```python
from build123d import *

# Parameters (mm, degrees)
F0_R           = 12.7
F1_DEPTH       = 60.325
F2_DEPTH       = 25.4
F4_DEPTH       = 19.05
F5_DEPTH       = 41.275
F6_R           = 5.08
F7_R           = 6.35
F8_DEPTH       = 25.4
F9_W           = 44.704
F9_H           = 22.3266
F10_DEPTH      = 25.4
F10_DEPTH_BACK = 25.4


with BuildPart() as f1:
    # F0 (on Front) → F1 (new body)
    with BuildSketch(Plane.XZ):
        with BuildLine():
            Line((36.865121601, 0.0010602231), (-26.6348784242, 0.0010602231))
            ThreePointArc((-26.6348784242, 0.0010602231), (-64.8692857058, 15.7277157318), (-48.7691742678, -22.3509397769))
            Line((-48.7691742678, -22.3509397769), (43.0772257322, -22.3509397769))
            Line((43.0772257322, -22.3509397769), (36.865121601, 0.0010602231))
        make_face()
        with Locations((-48.986878399, 0)):
            Circle(F0_R, mode=Mode.SUBTRACT)
        Polygon((68.259521601, 0.0010602231), (36.865121601, 0.0010602231), (43.0772257322, -22.3509397769), (68.4772257322, -22.3509397769), align=None)
        with BuildLine():
            ThreePointArc((82.5471727442, 34.7990602231), (78.7429689335, 16.0288506516), (68.259521601, 0.0010602231))
            Line((68.259521601, 0.0010602231), (101.101721601, 0.0010602231))
            Line((101.101721601, 0.0010602231), (101.101721601, 34.7990602231))
            Line((101.101721601, 34.7990602231), (82.5471727442, 34.7990602231))
        make_face()
        Polygon((101.101721601, 0.0010602231), (68.259521601, 0.0010602231), (68.4772257322, -22.3509397769), (145.4392257322, -22.3509397769), (145.4392257322, 0.0010602231), (145.2215215758, 0.0010602231), align=None)
    extrude(amount=F1_DEPTH)

    # F0 (on Front) → F2 (join)
    with BuildSketch(Plane.XZ):
        with BuildLine():
            Line((36.865121601, 0.0010602231), (-26.6348784242, 0.0010602231))
            ThreePointArc((-26.6348784242, 0.0010602231), (-64.8692857058, 15.7277157318), (-48.7691742678, -22.3509397769))
            Line((-48.7691742678, -22.3509397769), (43.0772257322, -22.3509397769))
            Line((43.0772257322, -22.3509397769), (36.865121601, 0.0010602231))
        make_face()
        with Locations((-48.986878399, 0)):
            Circle(F0_R, mode=Mode.SUBTRACT)
        Polygon((68.259521601, 0.0010602231), (36.865121601, 0.0010602231), (43.0772257322, -22.3509397769), (68.4772257322, -22.3509397769), align=None)
        with BuildLine():
            ThreePointArc((82.5471727442, 34.7990602231), (78.7429689335, 16.0288506516), (68.259521601, 0.0010602231))
            Line((68.259521601, 0.0010602231), (101.101721601, 0.0010602231))
            Line((101.101721601, 0.0010602231), (101.101721601, 34.7990602231))
            Line((101.101721601, 34.7990602231), (82.5471727442, 34.7990602231))
        make_face()
        Polygon((101.101721601, 0.0010602231), (68.259521601, 0.0010602231), (68.4772257322, -22.3509397769), (145.4392257322, -22.3509397769), (145.4392257322, 0.0010602231), (145.2215215758, 0.0010602231), align=None)
    extrude(amount=F2_DEPTH)

    # F3 (on face) → F4 (cut)
    with BuildSketch(Plane.XZ.offset(60.325)):
        Polygon((68.259521601, 0.0010602231), (36.865121601, 0.0010602231), (43.0772257322, -22.3509397769), (68.4772257322, -22.3509397769), align=None)
    extrude(amount=-F4_DEPTH, mode=Mode.SUBTRACT)

    # F0 (on Front) → F5 (cut)
    with BuildSketch(Plane.XZ):
        with BuildLine():
            ThreePointArc((82.5471727442, 34.7990602231), (78.7429689335, 16.0288506516), (68.259521601, 0.0010602231))
            Line((68.259521601, 0.0010602231), (101.101721601, 0.0010602231))
            Line((101.101721601, 0.0010602231), (101.101721601, 34.7990602231))
            Line((101.101721601, 34.7990602231), (82.5471727442, 34.7990602231))
        make_face()
    extrude(amount=F5_DEPTH, mode=Mode.SUBTRACT)

    # F6
    f6_edges = [f1.edges().sort_by_distance(p)[0] for p in [
        (101.101722, -50.8, 34.79906),
    ]]
    fillet(f6_edges, radius=F6_R)

    # F7 (on face) → F8 (cut)
    with BuildSketch(Plane.XY.offset(0.0010602231)):
        with Locations((106.5772257322, -22.352)):
            Circle(F7_R)
    extrude(amount=-F8_DEPTH, mode=Mode.SUBTRACT)

    # F9 (on Top) → F10 (cut, two sides)
    with BuildSketch(Plane.XY) as f10_sk:
        with Locations((-48.9868784242, -30.1625)):
            Rectangle(F9_W, F9_H)
    extrude(amount=F10_DEPTH, mode=Mode.SUBTRACT)
    extrude(f10_sk.sketch, amount=-F10_DEPTH_BACK, mode=Mode.SUBTRACT)


solid = f1.part
```
Source: CAD feature listing. Evaluate the final solid. Frame: model axes, mm. A direction names the side the tool comes from. Coordinates: 2 decimals unless noted, no trailing zeros. Loops run counter-clockwise (first coordinate to the right, second up) from the corner with the lowest first, then second, coordinate; pieces in that order, holes last. Notation, with made-up numbers: M 80,-22.5 L 117,-22.5 A28 cw 117,15.5 Z; hole C -23,56 d11. An arc over 180 degrees is marked long. Use CSV: the item, a comma, the result in double quotes.
(1) Cut plane D-D on x = 107. Return loops of the section in (y, z) (3 decimals).
Answers follow:
outline,"M -60.325,-22.351 L -28.688,-22.351 L -28.688,0.001 L -60.325,0.001 Z; M -16.016,-22.351 L 0,-22.351 L 0,0.001 L -16.016,0.001 Z"
(2) Line query: line 1 (Y direction, x = -32, z = -10) (3 decimals); line 2 (Z direction, x = 39, y = -24); line 3 (X direction, y = -45.5, z = 5). Output: solid intervals per line, ascending. Write a range as [from, to].
Answers follow:
line 1,"[-60.325, -41.326], [-18.999, 0]"
line 2,"[-22.35, 0]"
line 3,"[-70.77, -60.66], [-37.31, -27.2], [72.51, 101.1]"
(3) Cut plane A-A on y = -44.5. Return loops of the section in (x, z).
Answers follow:
outline,"M -48.77,-22.35 L 43.08,-22.35 L 36.87,0 L -26.63,0 A22.35 ccw long Z; M 68.26,0 L 68.48,-22.35 L 145.44,-22.35 L 145.44,0 L 101.1,0 L 101.1,29.72 A5.08 ccw 96.02,34.8 L 82.55,34.8 A50.8 cw Z; hole C -48.99,0 d25.4"
(4) Draft query along X for faces 1 (the face through (47, -30, -22.351)), 2 (the face through (78.845, -50.667, 16.279)), 3 (the face through (-59.065, -9.367, -7.728)), 4 (the face through (-64.341, -9.367, 16.244)). Return one class per face: pulls with the +X half, pulls with the -X half, needs draft (parallel to the pull), parting line crosses it, or undercut.
Answers follow:
face 1,"needs draft"
face 2,"undercut"
face 3,"undercut"
face 4,"parting line crosses it"
(5) Cut plane B-B on z = -8.5. Return loops of the section in (x, y) (3 decimals), and give its area (3 significant figures).
Answers follow:
outline,"M -69.66,-60.325 L -58.423,-60.325 L -58.423,-41.326 L -69.66,-41.326 Z; M -69.66,-18.999 L -58.423,-18.999 L -58.423,0 L -69.66,0 Z; M -39.551,-60.325 L 39.228,-60.325 L 39.228,-41.275 L 68.342,-41.275 L 68.342,-60.325 L 145.439,-60.325 L 145.439,0 L -39.551,0 L -39.551,-18.999 L -26.635,-18.999 L -26.635,-41.326 L -39.551,-41.326 Z; hole C 106.577,-22.352 d12.7"
area,"10,600 mm²"
(6) Cut plane C-C on z = 18. Return loops of the section in (x, y) (3 decimals).
Answers follow:
outline,"M -62.239,-60.325 L -35.735,-60.325 L -35.735,-41.326 L -62.239,-41.326 Z; M -62.239,-18.999 L -35.735,-18.999 L -35.735,0 L -62.239,0 Z; M 79.505,-60.325 L 101.102,-60.325 L 101.102,-41.275 L 79.505,-41.275 Z"
(7) Contact query for flat-ended pins moving along their axis: pin 1 (16.5 mm diameter, centred on x = 106.58, y = -22.35, fed in from +Z); pin 2 (23 mm diameter, centred on x = -48.99, z = 0, fed in from +Y); pin 3 (21 mm diameter, centred on y = -47.5, z = 17.5, fed in from +X); pin 4 (10 mm diameter, centred on x = 84.5, z = 24, fed in from +Y) (3 decimals). Output: stop coordinate, or through.
Answers follow:
pin 1,"z = 0"
pin 2,"through"
pin 3,"x = 101.1"
pin 4,"y = -41.275"
(8) Reachability of faces 5 (the face through (88, -41.275, 18)), 6 (the face through (101.102, -51, 15)), 7 (the face through (-39, -41.326, -10)) from +Z, -Z, +X, -X, +Y, -Y: full face, straight path, thin tool, end or side. Return the list, or none.
Answers follow:
face 5,"+Z, +X, -X, +Y"
face 6,"+Z, +X, +Y, -Y"
face 7,"+Z, -Z, -X"
